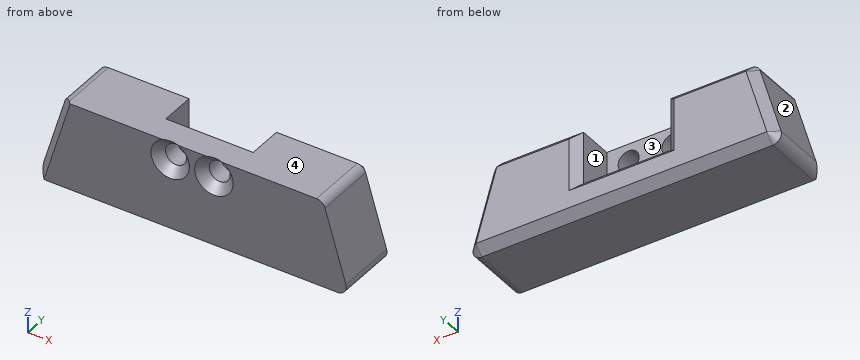
```python
from build123d import *

# Parameters (mm, degrees)
RESSALTO_EXTRUS_O2_DEPTH                             = 8
ESBO_O5_W                                            = 10
ESBO_O5_H                                            = 6
CORTE_EXTRUS_O1_DEPTH                                = 5
ESCAREADO_PARA_PARAFUSO_COM_CABE_A_ESCAR_D           = 2.4
ESCAREADO_PARA_PARAFUSO_COM_CABE_A_ESCAR_CSINK_D     = 4.4
ESCAREADO_PARA_PARAFUSO_COM_CABE_A_ESCAR_CSINK_ANGLE = 90
CHANFRO1_SIZE                                        = 1


with BuildPart() as part:
    # Esboço2 → Ressalto-extrusão2 (new body)
    with BuildSketch(Plane(origin=(0, 0, 0), x_dir=(1, 0, 0), z_dir=(0, 1, 0))):
        with BuildLine():
            Line((-0.213795634, 0.712652114), (-2.613795634, 8.712652114))
            ThreePointArc((-2.613795634, 8.712652114), (-2.458262277, 9.59693053), (-1.655969349, 10))
            Line((-1.655969349, 10), (31.655969349, 10))
            ThreePointArc((31.655969349, 10), (32.458262277, 9.59693053), (32.613795634, 8.712652114))
            Line((32.613795634, 8.712652114), (30.213795634, 0.712652114))
            ThreePointArc((30.213795634, 0.712652114), (29.852899879, 0.197707072), (29.255969349, 0))
            Line((29.255969349, 0), (0.744030651, 0))
            ThreePointArc((0.744030651, 0), (0.147100121, 0.197707072), (-0.213795634, 0.712652114))
        make_face()
    extrude(amount=RESSALTO_EXTRUS_O2_DEPTH)

    # Esboço5 → Corte-extrusão1 (cut)
    with BuildSketch(Plane(origin=(0, 8, 0), x_dir=(1, 0, 0), z_dir=(0, 1, 0))):
        with Locations((15, 3)):
            Rectangle(ESBO_O5_W, ESBO_O5_H)
    extrude(amount=-CORTE_EXTRUS_O1_DEPTH, mode=Mode.SUBTRACT)

    # Escareado para parafuso com cabeça escareada chata de M21 (through all)
    with Locations(Plane(origin=(17.5, 0, -2), x_dir=(0, 0, -1), z_dir=(0, -1, 0))):
        with Locations((0, 0), (0, -5)):
            CounterSinkHole(ESCAREADO_PARA_PARAFUSO_COM_CABE_A_ESCAR_D / 2, ESCAREADO_PARA_PARAFUSO_COM_CABE_A_ESCAR_CSINK_D / 2, counter_sink_angle=ESCAREADO_PARA_PARAFUSO_COM_CABE_A_ESCAR_CSINK_ANGLE)

    # Chanfro1
    # the kernel refuses this chamfer: 1 mm, written as the material it takes off along each edge
    with BuildSketch(Plane(origin=(10, 8, -6), x_dir=(0, 0, -1), z_dir=(1, 0, 0))) as chanfro1_piece_1:
        Polygon((CHANFRO1_SIZE, 0), (0, -CHANFRO1_SIZE), (0, 0), align=None)
    extrude(amount=10, mode=Mode.SUBTRACT)
    with BuildSketch(Plane(origin=(10, 8, 2.571682988), x_dir=(-1, 0, 0), z_dir=(0, 0, -1)), Plane(origin=(20, 8, -6), x_dir=(1, 0, 0), z_dir=(0, 0, 1))) as chanfro1_piece_2:
        Polygon((CHANFRO1_SIZE, 0), (0, -CHANFRO1_SIZE), (0, 0), align=None)
    extrude(amount=8.571682988, mode=Mode.SUBTRACT)
    with BuildSketch(Plane(origin=(12.571682988, 8, 0), x_dir=(0, 0, -1), z_dir=(-1, 0, 0)), Plane(origin=(29.255969349, 8, 0), x_dir=(0, 0, -1), z_dir=(-1, 0, 0))) as chanfro1_piece_3:
        Polygon((CHANFRO1_SIZE, 0), (0, CHANFRO1_SIZE), (0, 0), align=None)
    extrude(amount=11.827652337, mode=Mode.SUBTRACT)
    with BuildSketch(Plane(origin=(0.744030651, 8, -1), x_dir=(0, 0, 1), z_dir=(1, 0, 0))) as chanfro1_piece_4:
        Polygon((1 - CHANFRO1_SIZE, 0), (1, CHANFRO1_SIZE), (1, 0), align=None)
    revolve(axis=Axis((0.744030651, 8, -1), (0, -1, 0)), revolution_arc=73.300755766, mode=Mode.SUBTRACT)
    with BuildSketch(Plane(origin=(-0.213795634, 8, -0.712652114), x_dir=(0, -1, 0), z_dir=(-0.28734788556634544, 0, -0.9578262852211514))) as chanfro1_piece_5:
        Polygon((CHANFRO1_SIZE, 0), (0, -CHANFRO1_SIZE), (0, 0), align=None)
    extrude(amount=8.352245207, mode=Mode.SUBTRACT)
    with BuildSketch(Plane(origin=(-1.655969349, 8, -9), x_dir=(-0.957826285221151, 0, 0.2873478855663471), z_dir=(0.2873478855663471, 0, 0.957826285221151))) as chanfro1_piece_6:
        Polygon((1 - CHANFRO1_SIZE, 0), (1, CHANFRO1_SIZE), (1, 0), align=None)
    revolve(axis=Axis((-1.655969349, 8, -9), (0, -1, 0)), revolution_arc=106.699244234, mode=Mode.SUBTRACT)
    with BuildSketch(Plane(origin=(-1.655969349, 8, -10), x_dir=(0, 0, 1), z_dir=(1, 0, 0))) as chanfro1_piece_7:
        Polygon((CHANFRO1_SIZE, 0), (0, CHANFRO1_SIZE), (0, 0), align=None)
    extrude(amount=33.311938698, mode=Mode.SUBTRACT)
    with BuildSketch(Plane(origin=(31.655969349, 8, -9), x_dir=(0, 0, -1), z_dir=(-1, 0, 0))) as chanfro1_piece_8:
        Polygon((1 - CHANFRO1_SIZE, 0), (1, CHANFRO1_SIZE), (1, 0), align=None)
    revolve(axis=Axis((31.655969349, 8, -9), (0, -1, 0)), revolution_arc=106.699244234, mode=Mode.SUBTRACT)
    with BuildSketch(Plane(origin=(32.613795634, 8, -8.712652114), x_dir=(-0.9578262852211513, 0, -0.2873478855663455), z_dir=(-0.28734788556634555, 0, 0.9578262852211514))) as chanfro1_piece_9:
        Polygon((CHANFRO1_SIZE, 0), (0, CHANFRO1_SIZE), (0, 0), align=None)
    extrude(amount=8.352245207, mode=Mode.SUBTRACT)
    with BuildSketch(Plane(origin=(29.255969349, 8, -1), x_dir=(0.9578262852211534, 0, 0.2873478855663385), z_dir=(0.2873478855663385, 0, -0.9578262852211534))) as chanfro1_piece_10:
        Polygon((1 - CHANFRO1_SIZE, 0), (1, CHANFRO1_SIZE), (1, 0), align=None)
    revolve(axis=Axis((29.255969349, 8, -1), (0, -1, 0)), revolution_arc=73.300755766, mode=Mode.SUBTRACT)
    with BuildSketch(Plane(origin=(0.525172035, 0, 1.750573449), x_dir=(0, 1, 0), z_dir=(-0.28734788556634544, 0, -0.9578262852211514))) as chanfro1_piece_11:
        Polygon((CHANFRO1_SIZE, 0), (0, CHANFRO1_SIZE), (0, 0), align=None)
    extrude(amount=13.495611183, mode=Mode.SUBTRACT)
    with BuildSketch(Plane(origin=(10, 8, 0), x_dir=(-1, 0, 0), z_dir=(0, 0, -1))) as chanfro1_piece_12a_section:
        Polygon((CHANFRO1_SIZE, 0), (0, -CHANFRO1_SIZE), (0, 0), align=None)
    chanfro1_piece_12a = extrude(amount=8.571682988, mode=Mode.PRIVATE)
    chanfro1_piece_12a = split(chanfro1_piece_12a, bisect_by=Plane(origin=(10, 8, -6), z_dir=(0, 0, -1)), keep=Keep.TOP, mode=Mode.PRIVATE)
    with BuildSketch(Plane(origin=(7.428317012, 8, -6), x_dir=(0, 0, -1), z_dir=(1, 0, 0))) as chanfro1_piece_12b_section:
        Polygon((CHANFRO1_SIZE, 0), (0, -CHANFRO1_SIZE), (0, 0), align=None)
    chanfro1_piece_12b = extrude(amount=12.571682988, mode=Mode.PRIVATE)
    chanfro1_piece_12b = split(chanfro1_piece_12b, bisect_by=Plane(origin=(10, 8, -6), z_dir=(-1, 0, 0)), keep=Keep.TOP, mode=Mode.PRIVATE)
    chanfro1_piece_12 = chanfro1_piece_12a & chanfro1_piece_12b
    add(chanfro1_piece_12, mode=Mode.SUBTRACT)
    with BuildSketch(Plane(origin=(10, 8, -6), x_dir=(0, 0, -1), z_dir=(1, 0, 0))) as chanfro1_piece_13a_section:
        Polygon((CHANFRO1_SIZE, 0), (0, -CHANFRO1_SIZE), (0, 0), align=None)
    chanfro1_piece_13a = extrude(amount=12.571682988, mode=Mode.PRIVATE)
    chanfro1_piece_13a = split(chanfro1_piece_13a, bisect_by=Plane(origin=(20, 8, -6), z_dir=(1, 0, 0)), keep=Keep.TOP, mode=Mode.PRIVATE)
    with BuildSketch(Plane(origin=(20, 8, -8.571682988), x_dir=(1, 0, 0), z_dir=(0, 0, 1))) as chanfro1_piece_13b_section:
        Polygon((CHANFRO1_SIZE, 0), (0, -CHANFRO1_SIZE), (0, 0), align=None)
    chanfro1_piece_13b = extrude(amount=8.571682988, mode=Mode.PRIVATE)
    chanfro1_piece_13b = split(chanfro1_piece_13b, bisect_by=Plane(origin=(20, 8, -6), z_dir=(0, 0, -1)), keep=Keep.TOP, mode=Mode.PRIVATE)
    chanfro1_piece_13 = chanfro1_piece_13a & chanfro1_piece_13b
    add(chanfro1_piece_13, mode=Mode.SUBTRACT)


solid = part.part
```
Can you work these out from the model? Positions are in its coordinate system, mm. Face numbers are marked on the shaded views. Coordinates: 2 decimals unless noted, no trailing zeros. Loops run counter-clockwise (first coordinate to the right, second up) from the corner with the lowest first, then second, coordinate; pieces in that order, holes last. Notation, with made-up numbers: (29, 3) -> (58, 3) arc R13 ccw to (58, 15) -> close; hole circle Ø9 at (10.5, -12.5). An arc over 180 degrees is marked (long way). Answer as a JSON object with one key per item and string values.
1) Thinking about a two-plate mould opening in X: for the marked faces 1, 2, 3 and 4, which applies, pulls with the +X half, pulls with the -X half, needs draft (parallel to the pull), parting line crosses it, or undercut?
Results:
{"face 1": "undercut", "face 2": "pulls with the -X half", "face 3": "undercut", "face 4": "needs draft"}
2) Imagine slicing it at A-A (x = 12.5). Please give me the cut outline in (y, z).
Results:
{"outline": "(0, -10) -> (7, -10) -> (8, -9) -> (8, -7) -> (7, -6) -> (3, -6) -> (3, -3.2) -> (1, -3.2) -> (0, -4.2) -> close; (0.2, 0) -> (1, -0.8) -> (3, -0.8) -> (3, 0) -> close"}
3) Imagine slicing it at B-B (y = 1.5). Please give me the cut outline in (x, z).
Results:
{"outline": "(-2.61, -8.71) arc R1 ccw to (-1.66, -10) -> (31.66, -10) arc R1 ccw to (32.61, -8.71) -> (30.21, -0.71) arc R1 ccw to (29.26, 0) -> (0.74, 0) arc R1 ccw to (-0.21, -0.71) -> close; hole circle Ø2.4 at (12.5, -2); hole circle Ø2.4 at (17.5, -2)"}
4) Imagine slicing it at C-C (z = -2). Please give me the cut outline in (x, y), then the cut area to 3 significant figures.
Results:
{"outline": "(-0.6, 1) -> (0.44, 0) -> (10.3, 0) -> (11.3, 1) -> (11.3, 3) -> (10, 3) -> (10, 7) -> (9, 8) -> (0.44, 8) -> (-0.6, 7) -> close; (13.7, 1) -> (14.7, 0) -> (15.3, 0) -> (16.3, 1) -> (16.3, 3) -> (13.7, 3) -> close; (18.7, 1) -> (19.7, 0) -> (30.6, 0) -> (30.6, 7) -> (29.56, 8) -> (21, 8) -> (20, 7) -> (20, 3) -> (18.7, 3) -> close", "area": "181 mm^2"}
5) For P1, Ø3, axis at x = 12.5, z = -2, coming from the -Y side; P2, Ø3, axis at y = 4.5, z = -3.5, coming from the -X side; P3, Ø3, axis at x = 13, z = -1.5, coming from the +Y side, each with a flat end and sliding along its axis, tell me the tip position at first contact or that it passes through.
Results:
{"P1": "stops at y = 0.7", "P2": "stops at x = -1.5", "P3": "stops at y = 3"}
6) Imagine slicing it at D-D (y = 4.5). Please give me the cut outline in (x, z).
Results:
{"outline": "(-2.61, -8.71) arc R1 ccw to (-1.66, -10) -> (31.66, -10) arc R1 ccw to (32.61, -8.71) -> (30.21, -0.71) arc R1 ccw to (29.26, 0) -> (20, 0) -> (20, -6) -> (10, -6) -> (10, 0) -> (0.74, 0) arc R1 ccw to (-0.21, -0.71) -> close"}
7) If I drill on line 1 (X direction, y = 1.5, z = -2.5); line 2 (Z direction, x = 17.5, y = 2.4); line 3 (X direction, y = 2.25, z = -2), over which ranges is the centre line in solid material (lowest first)?
Results:
{"line 1": "x = -0.75 to 11.41, 13.59 to 16.41, 18.59 to 30.75", "line 2": "z = -10 to -3.2, -0.8 to 0", "line 3": "x = -0.6 to 11.3, 13.7 to 16.3, 18.7 to 30.6"}
